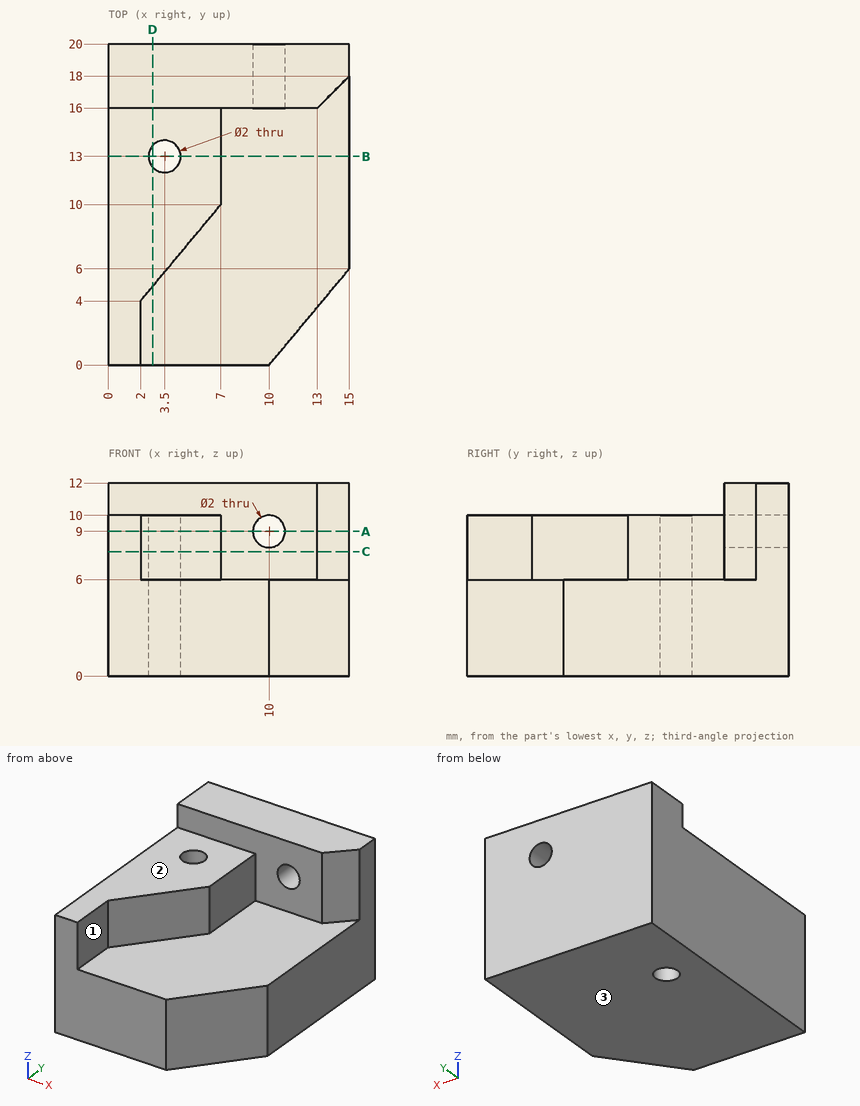
The figure shows three views and two pictorial views of one solid part (mm, origin at its lowest corner). Answer the questions. A direction names the side the tool comes from. Coordinates: 2 decimals unless noted, no trailing zeros. Order: outer loops, then holes, each group sorted by start corner. A loop starts at its lowest first (then second) coordinate and runs counter-clockwise, first axis right, second up.
Q1. Given P1, Ø1.5, axis at x = 6, y = 8.5, coming from the +Z side; P2, Ø4, axis at x = 12.5, y = 13, coming from the +Z side; P3, Ø2, axis at y = 1.5, z = 8.5, coming from the +X side, each flat-ended and moving along its own axis, determine where each tip first touches the part or whether it passes through.
Q2. A cutting plane is placed at C-C, the plane z = 7.75. Write down the section's boundary in (x, y).
Q3. A cutting plane is placed at D-D, the plane x = 2.75. Write down the section's boundary in (y, z).
Q4. Which of the six approach directions +Z, -Z, +X, -X, +Y, -Y give full straight-line access (tool end or side, diameter ignored) to the marked faces 1, 2 and 3?
Q5. A cutting plane is placed at B-B, the plane y = 13. Write down the section's boundary in (x, z).
Q6. Consider line 1 (Y direction, x = 3.5, z = 4.75); line 2 (X direction, y = 13, z = 4.25); line 3 (Z direction, x = 5.25, y = 1.25). Determine where each line is inside the solid, lowest interval first.
Q7. A cutting plane is placed at A-A, the plane z = 9. Write down the section's boundary in (x, y).
Answers follow:
1. P1: stops at z = 10
1. P2: stops at z = 6
1. P3: stops at x = 2
2. outline: (0, 0) - (2, 0) - (2, 4) - (7, 10) - (7, 16) - (13, 16) - (15, 18) - (15, 20) - (0, 20) - close; hole circle Ø2 at (3.5, 13)
3. outline: (0, 0) - (12.34, 0) - (12.34, 10) - (4.9, 10) - (4.9, 6) - (0, 6) - close; (13.66, 0) - (20, 0) - (20, 12) - (16, 12) - (16, 10) - (13.66, 10) - close
4. face 1: +Z, +X, -Y
4. face 2: +Z, +X, -X, -Y
4. face 3: -Z, +X, -X, +Y, -Y
5. outline: (0, 0) - (2.5, 0) - (2.5, 10) - (0, 10) - close; (4.5, 0) - (15, 0) - (15, 6) - (7, 6) - (7, 10) - (4.5, 10) - close
6. line 1: y = 0 to 12, 14 to 20
6. line 2: x = 0 to 2.5, 4.5 to 15
6. line 3: z = 0 to 6
7. outline: (0, 0) - (2, 0) - (2, 4) - (7, 10) - (7, 16) - (9, 16) - (9, 20) - (0, 20) - close; (11, 16) - (13, 16) - (15, 18) - (15, 20) - (11, 20) - close; hole circle Ø2 at (3.5, 13)
